Study the drawing (mm; zero at the part's minimum x, y, z) and answer. Give positions to 0.01 mm unless a question says otherwise; leave off trailing zeros. Order: outer loops, then holes, each group sorted by start corner. A loop starts at its lowest first (then second) coordinate and runs counter-clockwise, first axis right, second up. Notation, with made-up numbers: (19, -34) - (52, -34) arc R23 cw to (52, -26) - close; hole circle Ø9 at (71.5, 81.25). An arc over 180 degrees is marked (long way). Write each question's results on one line, items separated by ' | '. Start each with the question number.
1. Section A-A (y = 6) is taken. Give the vertices of the cut face in (x, z).
2. A flat-ended cylindrical pin translates along its axis: pin 1 (3.5 mm diameter, centred on y = 6, z = 189, fed in from +X). Find the tip coordinate at first contact, or state that the pin passes through.
3. Find the intervals of material crossed by L1, parallel to Z at x = 3.75, y = 6; L2, parallel to Z at x = 3.25, y = 6; L3, parallel to Y at x = 7, z = 189, in increasing order.
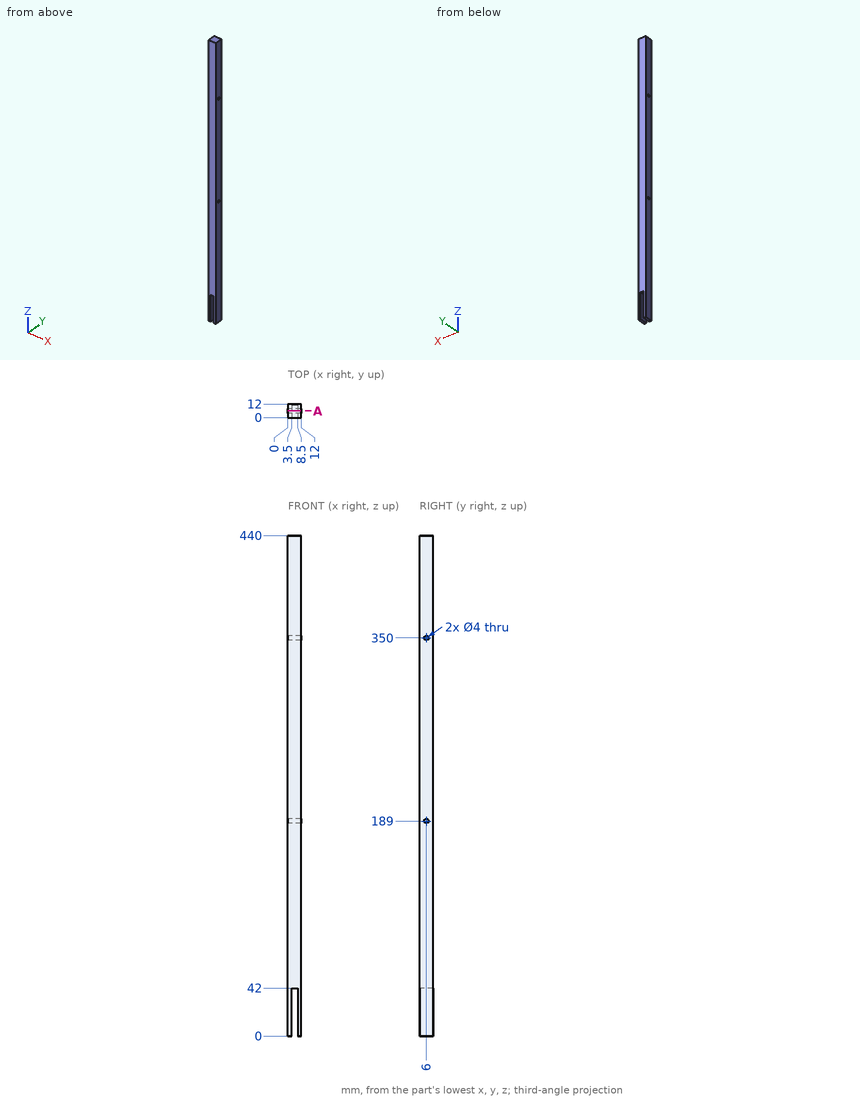
Reported:
1) outline: (0, 0) - (3.5, 0) - (3.5, 42) - (8.5, 42) - (8.5, 0) - (12, 0) - (12, 187) - (0, 187) - close; (0, 191) - (12, 191) - (12, 348) - (0, 348) - close; (0, 352) - (12, 352) - (12, 440) - (0, 440) - close
2) pin 1: through
3) L1: 42 to 187, 191 to 348, 352 to 440 | L2: 0 to 187, 191 to 348, 352 to 440 | L3: 0 to 4, 8 to 12
